Design review of the part built by this model. Coordinates are the model's own, in mm. A direction names the side the tool comes from. Coordinates: 2 decimals unless noted, no trailing zeros. Loops run counter-clockwise (first coordinate to the right, second up) from the corner with the lowest first, then second, coordinate; pieces in that order, holes last. Notation, with made-up numbers: (36, 25) -> (89, 25) arc R14 cw to (89, 39) -> close; hole circle Ø1 at (83.5, 87.25). An arc over 180 degrees is marked (long way). Answer in a Markdown table with one row per item.
```python
from build123d import *

# Parameters (mm, degrees)
BOSS_EXTRUDE1_DEPTH = 5
SKETCH1_3_W         = 15
SKETCH1_3_H         = 1
BOSS_EXTRUDE2_DEPTH = 10
BOSS_EXTRUDE3_START = 5
SKETCH1_4_R         = 0.675
BOSS_EXTRUDE3_DEPTH = 2.5


with BuildPart() as part:
    # Sketch1 → Boss-Extrude1 (new body)
    with BuildSketch(Plane.XY):
        with BuildLine():
            Line((-34.696792319, 15.960080691), (-34.696792319, 14.960080691))
            Line((-34.696792319, 14.960080691), (-19.696792319, 14.960080691))
            ThreePointArc((-19.696792319, 14.960080691), (-8.978328635, 10.128349866), (-4.442261745, -0.718547556))
            ThreePointArc((-4.442261745, -0.718547556), (0.138348196, -4.497872806), (4.478025356, -0.444172161))
            ThreePointArc((4.478025356, -0.444172161), (-9.240182202, 21.774129955), (-34.696792319, 15.960080691))
        make_face()
        with BuildLine():
            Line((-3.89291928, 2.43426562), (-7.593303854, 13.845333863))
            ThreePointArc((-7.593303854, 13.845333863), (-6.157572873, 16.914026296), (-3.083690723, 15.489440313))
            Line((-3.083690723, 15.489440313), (1.566927521, 4.392862954))
            Line((1.566927521, 4.392862954), (1.798943002, 3.572646648))
            ThreePointArc((1.798943002, 3.572646648), (1.351572105, -3.764738085), (-3.660510182, 1.612657808))
            Line((-3.660510182, 1.612657808), (-3.89291928, 2.43426562))
        make_face(mode=Mode.SUBTRACT)
    extrude(amount=BOSS_EXTRUDE1_DEPTH)

    # Sketch1<3> → Boss-Extrude2 (add)
    with BuildSketch(Plane.XY):
        with Locations((-27.196792319, 15.460080691)):
            Rectangle(SKETCH1_3_W, SKETCH1_3_H)
    extrude(amount=BOSS_EXTRUDE2_DEPTH)

    # Sketch1<4> → Boss-Extrude3 (add)
    with BuildSketch(Plane.XY.offset(BOSS_EXTRUDE3_START)):
        with BuildLine():
            Line((1.622209226, 4.197432218), (1.566927521, 4.392862954))
            Line((1.566927521, 4.392862954), (-3.083690723, 15.489440313))
            ThreePointArc((-3.083690723, 15.489440313), (-6.157572873, 16.914026296), (-7.593303854, 13.845333863))
            Line((-7.593303854, 13.845333863), (-3.89291928, 2.43426562))
            Line((-3.89291928, 2.43426562), (-3.859078085, 2.314630929))
            ThreePointArc((-3.859078085, 2.314630929), (-3.110655329, 3.251741598), (-2.141289558, 3.957888203))
            ThreePointArc((-2.141289558, 3.957888203), (-1.804156256, 4.956878575), (-0.903758531, 4.408312661))
            ThreePointArc((-0.903758531, 4.408312661), (0.374380142, 4.484399571), (1.622209226, 4.197432218))
        make_face()
        with Locations((-5.335514236, 14.659204884)):
            Circle(SKETCH1_4_R, mode=Mode.SUBTRACT)
        with Locations((-3.830625605, 10.524557353)):
            Circle(SKETCH1_4_R, mode=Mode.SUBTRACT)
        with Locations((-4.583069921, 12.591881119)):
            Circle(SKETCH1_4_R, mode=Mode.SUBTRACT)
        with Locations((-2.325736975, 6.389909821)):
            Circle(SKETCH1_4_R, mode=Mode.SUBTRACT)
        with Locations((-3.07818129, 8.457233587)):
            Circle(SKETCH1_4_R, mode=Mode.SUBTRACT)
    extrude(amount=-BOSS_EXTRUDE3_DEPTH)


solid = part.part
```
(1) To check wall thickness, follow probe 1 along Y at (x, z) = (-26.5, 5.5); probe 2 along Z at (x, y) = (-9.5, 18.75); probe 3 along Y at (x, z) = (0, 1.35). State the ranges of each line that lie inside material, in increasing order.
Evaluation:
| item | result |
|---|---|
| probe 1 | y = 14.96 to 15.96 |
| probe 2 | z = 0 to 5 |
| probe 3 | y = -4.5 to -4, 8.13 to 14.6 |
(2) Take a section at C-C on z = 6.25. Give the boundary of the cut face in (x, y).
Evaluation:
| item | result |
|---|---|
| outline | (-34.7, 14.96) -> (-19.7, 14.96) -> (-19.7, 15.96) -> (-34.7, 15.96) -> close |
(3) Draft analysis for pull direction Y (two halves, no side actions). For faces 1 (the cylindrical face through (-3.166, 9.126, 3.768)), 2 (the flat face through (-11, 16, 5)), 3 (the cylindrical face through (0, -4.5, 2.5)), state which applies: pulls with the +Y half, pulls with the -Y half, needs draft (parallel to the pull), parting line crosses it, or undercut.
Evaluation:
| item | result |
|---|---|
| face 1 | undercut |
| face 2 | needs draft |
| face 3 | pulls with the -Y half |
(4) Take a section at A-A on y = 0. Give the boundary of the cut face in (x, z).
Evaluation:
| item | result |
|---|---|
| outline | (-4.47, 0) -> (-4, 0) -> (-4, 5) -> (-4.47, 5) -> close; (4, 0) -> (4.5, 0) -> (4.5, 5) -> (4, 5) -> close |
(5) Take a section at D-D on x = -16. Give the boundary of the cut face in (y, z), and give its area (3 significant figures).
Evaluation:
| item | result |
|---|---|
| outline | (14.34, 0) -> (23.43, 0) -> (23.43, 5) -> (14.34, 5) -> close |
| area | 45.5 mm² |
(6) Tool access review of faces 4 (the flat face through (-5.717, 8.06, 1.232)), 5 (the flat face through (-27, 14.96, 5)), 6 (the cylindrical face through (0.356, 4.486, 3.768)): name each direction out of +Z, -Z, +X, -X, +Y, -Y from which nothing blocks a thin tool from reaching the whole face with its end or side.
Evaluation:
| item | result |
|---|---|
| face 4 | -Z |
| face 5 | +Z, -Z, -X, -Y |
| face 6 | +Z, -Z |
(7) Take a section at B-B on x = 0. Give the boundary of the cut face in (y, z), and give its area (3 significant figures).
Evaluation:
| item | result |
|---|---|
| outline | (-4.5, 0) -> (-4, 0) -> (-4, 5) -> (-4.5, 5) -> close; (4.5, 2.5) -> (8.13, 2.5) -> (8.13, 0) -> (14.6, 0) -> (14.6, 5) -> (4.5, 5) -> close |
| area | 43.9 mm² |
(8) For pin 1 (10.5 mm diameter, centred on x = 0, y = 0, fed in from +Z); pin 2 (4 mm diameter, centred on x = -27, z = 8, fed in from +Y); pin 3 (1.8 mm diameter, centred on x = -3.83, y = 10.52, fed in from -Z), all flat-tipped, find the tip position at first contact; note any pin that passes through.
Evaluation:
| item | result |
|---|---|
| pin 1 | stops at z = 5 |
| pin 2 | stops at y = 15.96 |
| pin 3 | stops at z = 2.5 |
